Part model, mm, in its own coordinate system. Round coordinates to 2 decimals unless told otherwise and drop trailing zeros. Write each loop counter-clockwise with the first axis right and the second up, starting at its lowest first coordinate (ties: lowest second). Pieces come first, ordered by that corner, then holes.
1) Saw through at A-A on y = -4. Write the cut outline in (x, z).
2) Saw through at B-B on x = 21. Write the cut outline in (y, z), and give its area (3 significant figures).
3) Saw through at D-D on y = -54. Write the cut outline in (x, z), and give its area (3 significant figures).
4) Pull direction X, two halves, no side cores. Call faces 1 (the flat face through (1, -141, 2)), 2 (the cylindrical face through (15.741, 14.475, 0.986)), 3 (the cylindrical face through (-10.5, -100.4, 1)): +X half, -X half, draft (parallel to the pull), parting line (faces both ways), or undercut.
5) Flat gauge pins, fed straight in: pin 1 (4 mm diameter, centred on x = 15, y = -59, fed in from -Z) (1 decimal); pin 2 (1 mm diameter, centred on y = -143, z = 1, fed in from +X). Where does each tip first touch, or does it go through?
6) Drill centre lines: L1, parallel to Y at x = 0, z = 1; L2, parallel to Y at x = -32.5, z = 1.5; L3, parallel to Y at x = 3.5, z = 1.75. Where is each one in solid material? Low to high.
7) Saw through at C-C on z = 0.6. Count the separate pieces of the cut face and the enclosed holes in it, and give its area (3 significant figures).
```python
from build123d import *

# Parameters (mm, degrees)
SKETCH_3_R      = 2
SKETCH_3_R_2    = 1.5
SKETCH_3_R_3    = 24
SKETCH_3_R_4    = 15
SKETCH_3_R_5    = 9.300530536
SKETCH_3_R_6    = 6.764022208
EXTRUDE_1_DEPTH = 2


with BuildPart() as part:
    # 草图3 → 凸台-拉伸1 (new body)
    with BuildSketch(Plane.XY):
        with BuildLine():
            Line((-45.000000203, -253.990216873), (-45.000000203, -225.990216873))
            ThreePointArc((-45.000000203, -225.990216873), (-10.464636425, -98.498581931), (-41.000000203, 30.00978313))
            ThreePointArc((-41.000000203, 30.00978313), (-34.337300158, 30.272772604), (-28.47422393, 27.097072286))
            ThreePointArc((-28.47422393, 27.097072286), (-27.224139288, 25.786699845), (-25.913815771, 24.536563921))
            ThreePointArc((-25.913815771, 24.536563921), (-15.930569702, 14.552804479), (-1.811764705, 14.5524367))
            ThreePointArc((-1.811764705, 14.5524367), (-0.001002499, 14.509783327), (1.809761926, 14.552342399))
            ThreePointArc((1.809761926, 14.552342399), (15.928572681, 14.55197476), (25.912339468, 24.535221628))
            ThreePointArc((25.912339468, 24.535221628), (27.223433456, 25.78599462), (28.474223558, 27.097072286))
            ThreePointArc((28.474223558, 27.097072286), (34.337299786, 30.272772604), (40.999999832, 30.00978313))
            ThreePointArc((40.999999832, 30.00978313), (10.464636053, -98.498581931), (44.999999832, -225.990216873))
            Line((44.999999832, -225.990216873), (44.999999832, -253.990216873))
            Line((44.999999832, -253.990216873), (40.999999832, -253.990216873))
            Line((40.999999832, -253.990216873), (25.699999832, -253.990216873))
            Line((25.699999832, -253.990216873), (25.699999832, -249.890216873))
            Line((25.699999832, -249.890216873), (25.699999832, -248.890216873))
            Line((25.699999832, -248.890216873), (12.699999797, -248.890216873))
            Line((12.699999797, -248.890216873), (12.699999797, -245.890216873))
            Line((12.699999797, -245.890216873), (-12.700000168, -245.890216873))
            Line((-12.700000168, -245.890216873), (-12.700000168, -248.890216873))
            Line((-12.700000168, -248.890216873), (-25.700000203, -248.890216873))
            Line((-25.700000203, -248.890216873), (-25.700000203, -249.890216873))
            Line((-25.700000203, -249.890216873), (-25.700000203, -253.990216873))
            Line((-25.700000203, -253.990216873), (-41.000000203, -253.990216873))
            Line((-41.000000203, -253.990216873), (-42, -253.990216873))
            Line((-42, -253.990216873), (-44.000000203, -253.990216873))
            Line((-44.000000203, -253.990216873), (-45.000000203, -253.990216873))
        make_face()
        with Locations((0, 10.509783315)):
            Circle(SKETCH_3_R, mode=Mode.SUBTRACT)
        with Locations((-30.0520382, 22.957745114)):
            Circle(SKETCH_3_R, mode=Mode.SUBTRACT)
        with Locations((30.0520382, 22.957745114)):
            Circle(SKETCH_3_R, mode=Mode.SUBTRACT)
        with Locations((41.999999628, -239.990216688)):
            Circle(SKETCH_3_R_2, mode=Mode.SUBTRACT)
        with Locations(Location((-42, -239.990216688, 0), (0, 0, 180))):
            Circle(SKETCH_3_R_2, mode=Mode.SUBTRACT)
        with Locations((0, -212.7618397)):
            Circle(SKETCH_3_R_3, mode=Mode.SUBTRACT)
        with Locations((0, -9.975031617)):
            Circle(SKETCH_3_R_4, mode=Mode.SUBTRACT)
        with Locations((0, -162.250886598)):
            Circle(SKETCH_3_R_5, mode=Mode.SUBTRACT)
        with Locations((0, -38.807481302)):
            Circle(SKETCH_3_R_6, mode=Mode.SUBTRACT)
        with BuildLine():
            Line((-37.1, -252.090216688), (-29.9, -252.090216688))
            Line((-29.9, -252.090216688), (-29.9, -249.890216688))
            Line((-29.9, -249.890216688), (-37.1, -249.890216688))
            ThreePointArc((-37.1, -249.890216688), (-37.555634919, -250.990216688), (-37.1, -252.090216688))
        make_face(mode=Mode.SUBTRACT)
        with BuildLine():
            Line((29.9, -252.090216688), (29.9, -249.890216688))
            Line((29.9, -249.890216688), (37.1, -249.890216688))
            ThreePointArc((37.1, -249.890216688), (37.555634919, -250.990216688), (37.1, -252.090216688))
            Line((37.1, -252.090216688), (29.9, -252.090216688))
        make_face(mode=Mode.SUBTRACT)
        with BuildLine():
            Line((-43.1, -244.890216688), (-43.1, -250.090216688))
            Line((-43.1, -250.090216688), (-40.9, -250.090216688))
            Line((-40.9, -250.090216688), (-40.9, -244.890216688))
            ThreePointArc((-40.9, -244.890216688), (-42, -244.434581769), (-43.1, -244.890216688))
        make_face(mode=Mode.SUBTRACT)
        with BuildLine():
            Line((-43.1, -229.890216688), (-43.1, -235.090216688))
            ThreePointArc((-43.1, -235.090216688), (-42, -235.545851606), (-40.9, -235.090216688))
            Line((-40.9, -235.090216688), (-40.9, -229.890216688))
            Line((-40.9, -229.890216688), (-43.1, -229.890216688))
        make_face(mode=Mode.SUBTRACT)
        with BuildLine():
            Line((40.899999628, -229.890216688), (40.899999628, -235.090216688))
            ThreePointArc((40.899999628, -235.090216688), (41.999999628, -235.545851606), (43.099999628, -235.090216688))
            Line((43.099999628, -235.090216688), (43.099999628, -229.890216688))
            Line((43.099999628, -229.890216688), (40.899999628, -229.890216688))
        make_face(mode=Mode.SUBTRACT)
        with BuildLine():
            Line((40.899999628, -244.890216688), (40.899999628, -250.090216688))
            Line((40.899999628, -250.090216688), (43.099999628, -250.090216688))
            Line((43.099999628, -250.090216688), (43.099999628, -244.890216688))
            ThreePointArc((43.099999628, -244.890216688), (41.999999628, -244.434581769), (40.899999628, -244.890216688))
        make_face(mode=Mode.SUBTRACT)
    extrude(amount=EXTRUDE_1_DEPTH)


solid = part.part
```
Completed:
1. outline: (-26.1, 0) - (-13.76, 0) - (-13.76, 2) - (-26.1, 2) - close; (13.76, 0) - (26.1, 0) - (26.1, 2) - (13.76, 2) - close
2. outline: (-248.89, 0) - (-224.38, 0) - (-224.38, 2) - (-248.89, 2) - close; (-201.14, 0) - (-168.84, 0) - (-168.84, 2) - (-201.14, 2) - close; (-19.78, 0) - (17.7, 0) - (17.7, 2) - (-19.78, 2) - close
2. area: 189 mm2
3. outline: (-13.48, 0) - (13.48, 0) - (13.48, 2) - (-13.48, 2) - close
3. area: 53.9 mm2
4. face 1: draft
4. face 2: undercut
4. face 3: -X half
5. pin 1: passes through
5. pin 2: stops at x = 14.98
6. L1: y = -245.89 to -236.76, -188.76 to -171.55, -152.95 to -45.57, -32.04 to -24.98, 5.02 to 8.51, 12.51 to 14.51
6. L2: y = -253.99 to -252.09, -249.89 to -200.82, 12.2 to 29.69
6. L3: y = -245.89 to -236.51, -189.02 to -170.87, -153.63 to -44.6, -33.02 to -24.56, 4.61 to 13.95
7. separate pieces: 1
7. enclosed holes: 15
7. area: 9,100 mm2
